```python
from build123d import *

# Parameters (mm, degrees)
SKETCH_1_W      = 23
SKETCH_1_H      = 23
SKETCH_1_R      = 1.5
SKETCH_1_R_2    = 6.5
EXTRUDE_1_DEPTH = 1
FILLET_1_R      = 1


with BuildPart() as part:
    # 草图1 → 凸台-拉伸1 (new body)
    with BuildSketch(Plane.XY):
        Rectangle(SKETCH_1_W, SKETCH_1_H)
        with Locations((-8.838834765, 8.838834765)):
            Circle(SKETCH_1_R, mode=Mode.SUBTRACT)
        with Locations(Location((-8.838834765, -8.838834765, 0), (0, 0, 180))):
            Circle(SKETCH_1_R, mode=Mode.SUBTRACT)
        with Locations((8.838834765, -8.838834765)):
            Circle(SKETCH_1_R, mode=Mode.SUBTRACT)
        with Locations(Location((8.838834765, 8.838834765, 0), (0, 0, 180))):
            Circle(SKETCH_1_R, mode=Mode.SUBTRACT)
        Circle(SKETCH_1_R_2, mode=Mode.SUBTRACT)
    extrude(amount=EXTRUDE_1_DEPTH)

    # 圆角1
    fillet_1_edges = [part.edges().sort_by_distance(p)[0] for p in [
        (-11.5, 11.5, 0.5),
        (11.5, 11.5, 0.5),
        (11.5, -11.5, 0.5),
        (-11.5, -11.5, 0.5),
    ]]
    fillet(fillet_1_edges, radius=FILLET_1_R)


solid = part.part
```
For this review, take the finished solid that the model builds, in its own axes (mm). Round coordinates to 2 decimals unless told otherwise and drop trailing zeros. Order: outer loops, then holes, each group sorted by start corner. A loop starts at its lowest first (then second) coordinate and runs counter-clockwise, first axis right, second up.
Q1. We need section D-D, the plane z = 0.25. Give the boundary of the cut face in (x, y), plus the area to 3 significant figures.
Findings below:
outline: (-11.5, -10.5) arc R1 ccw to (-10.5, -11.5) - (10.5, -11.5) arc R1 ccw to (11.5, -10.5) - (11.5, 10.5) arc R1 ccw to (10.5, 11.5) - (-10.5, 11.5) arc R1 ccw to (-11.5, 10.5) - close; hole circle Ø3 at (-8.84, -8.84); hole circle Ø3 at (-8.84, 8.84); hole circle Ø13 at (0, 0); hole circle Ø3 at (8.84, -8.84); hole circle Ø3 at (8.84, 8.84)
area: 367 mm2
Q2. Wall thickness on line 1 (Y direction, x = -8.5, z = 0.9); line 2 (Y direction, x = 0, z = 0.4); line 3 (Y direction, x = -2, z = 0.45): over which ranges is each line inside the solid? List them lowest first.
Findings below:
line 1: y = -11.5 to -10.3, -7.38 to 7.38, 10.3 to 11.5
line 2: y = -11.5 to -6.5, 6.5 to 11.5
line 3: y = -11.5 to -6.18, 6.18 to 11.5
Q3. We need section A-A, the plane y = 0. Give the boundary of the cut face in (x, z), plus the area to 3 significant figures.
Findings below:
outline: (-11.5, 0) - (-6.5, 0) - (-6.5, 1) - (-11.5, 1) - close; (6.5, 0) - (11.5, 0) - (11.5, 1) - (6.5, 1) - close
area: 10.0 mm2
Q4. We need section C-C, the plane x = 9.5. Give the boundary of the cut face in (y, z).
Findings below:
outline: (-11.5, 0) - (-10.19, 0) - (-10.19, 1) - (-11.5, 1) - close; (-7.49, 0) - (7.49, 0) - (7.49, 1) - (-7.49, 1) - close; (10.19, 0) - (11.5, 0) - (11.5, 1) - (10.19, 1) - close
Q5. Mouldability with a two-part tool opening along Y and no side actions: class faces 1 (the cylindrical face through (-5.158, -3.955, 0.493)), 2 (the cylindrical face through (-10.03, 7.93, 0.49)), 3 (the flat face through (5, -5, 0)), 4 (the cylindrical face through (-11.215, 11.199, 0.507)) as pulls with the +Y half, pulls with the -Y half, needs draft (parallel to the pull), parting line crosses it, or undercut.
Findings below:
face 1: undercut
face 2: undercut
face 3: needs draft
face 4: pulls with the +Y half
Q6. Insertion check: P1, Ø5, axis at x = 7.5, y = 0, coming from the -Z side. The pin has a flat end and moves straight along its axis. Give the tip position at first contact, or say it passes through.
Findings below:
P1: stops at z = 0
